Input: part model. Units: mm. Frame: model coordinates. A direction names the side the tool comes from. Round coordinates to 2 decimals unless told otherwise and drop trailing zeros. Loops run counter-clockwise (first coordinate to the right, second up) from the corner with the lowest first, then second, coordinate; pieces in that order, holes last. Notation, with made-up numbers: (3.5, -24.5) -> (36.5, -24.5) arc R19 ccw to (36.5, -10.5) -> close; hole circle Ø4 at (45.25, -19). An arc over 180 degrees is marked (long way). Answer as a JSON object with one key per item and string values. Group by question number.
Item 1: Section query B-B on z = 10. Return loops of the section in (x, y).
Item 2: Section query A-A on x = 0. Return loops of the section in (y, z), and give its area (3 significant figures).
Item 3: Section query C-C on y = -14. Return loops of the section in (x, z), and give its area (3 significant figures).
Item 4: Set-up query: faces 4 (the cylindrical face through (0.51, -74.23, -8.38)), 5 (the flat face through (-2, 72.2, 9)), 6 (the flat face through (-2, -72.2, -9)). Return all of +Z, -Z, +X, -X, +Y, -Y with unobstructed straight access to the full face (end or side cutting, diameter ignored); none if empty.
Item 5: Pin query (flat end, axial travel): pin 1 (1 mm diameter, centred on x = 5.5, y = -6.5, fed in from +Z); pin 2 (2.5 mm diameter, centred on x = -0.5, z = 9.5, fed in from +Y); pin 3 (5 mm diameter, centred on x = -4.5, y = -27, fed in from -Z). Return the tip coordinate at first contact, or that it passes through.
Item 6: Material intervals for line 1 (Y direction, x = 3.5, z = 7.75); line 2 (X direction, y = 74.35, z = 10); line 3 (Z direction, x = -0.25, y = -47), sorted ascending. Write a range as [from, to].
Item 7: Draft query along Z for faces 1 (the flat face through (0, -74, -13.75)), 2 (the cylindrical face through (-1.66, 74.23, 9.63)), 3 (the flat face through (-7, 0, 1)). Return one class per face: released by +Z, released by -Z, zero draft, split by the parting line, or undercut.
from build123d import *

# Parameters (mm, degrees)
SKETCH1_W           = 14
SKETCH1_H           = 10
BOSS_EXTRUDE1_DEPTH = 76.2
SKETCH3_W           = 14
SKETCH3_H           = 27.5
SKETCH3_R           = 1.7
BOSS_EXTRUDE3_DEPTH = 4


with BuildPart() as part:
    # Sketch1 → Boss-Extrude1 (new, symmetric)
    with BuildSketch(Plane(origin=(0, 0, 0), x_dir=(1, 0, 0), z_dir=(0, 1, 0))):
        Rectangle(SKETCH1_W, SKETCH1_H)
    extrude(amount=BOSS_EXTRUDE1_DEPTH, both=True)

    # Sketch3 → Boss-Extrude3 (add)
    with BuildSketch(Plane(origin=(0, 76.2, 0), x_dir=(1, 0, 0), z_dir=(0, 1, 0))):
        Rectangle(SKETCH3_W, SKETCH3_H)
        with Locations(Location((0, 10, 0), (0, 0, 270))):
            Circle(SKETCH3_R, mode=Mode.SUBTRACT)
        with Locations(Location((0, -10, 0), (0, 0, 270))):
            Circle(SKETCH3_R, mode=Mode.SUBTRACT)
    boss_extrude3 = extrude(amount=-BOSS_EXTRUDE3_DEPTH)

    # Mirror1: Boss-Extrude3 across plane
    add(boss_extrude3.mirror(Plane.ZX))


solid = part.part
Solved:
{
 "1": {"outline": "(-7, -76.2) -> (-1.7, -76.2) -> (-1.7, -72.2) -> (-7, -72.2) -> close; (-7, 72.2) -> (-1.7, 72.2) -> (-1.7, 76.2) -> (-7, 76.2) -> close; (1.7, -76.2) -> (7, -76.2) -> (7, -72.2) -> (1.7, -72.2) -> close; (1.7, 72.2) -> (7, 72.2) -> (7, 76.2) -> (1.7, 76.2) -> close"},
 "2": {"outline": "(-76.2, -13.75) -> (-72.2, -13.75) -> (-72.2, -11.7) -> (-76.2, -11.7) -> close; (-76.2, -8.3) -> (-72.2, -8.3) -> (-72.2, -5) -> (72.2, -5) -> (72.2, -8.3) -> (76.2, -8.3) -> (76.2, 8.3) -> (72.2, 8.3) -> (72.2, 5) -> (-72.2, 5) -> (-72.2, 8.3) -> (-76.2, 8.3) -> close; (-76.2, 11.7) -> (-72.2, 11.7) -> (-72.2, 13.75) -> (-76.2, 13.75) -> close; (72.2, -13.75) -> (76.2, -13.75) -> (76.2, -11.7) -> (72.2, -11.7) -> close; (72.2, 11.7) -> (76.2, 11.7) -> (76.2, 13.75) -> (72.2, 13.75) -> close", "area": "1,610 mm²"},
 "3": {"outline": "(-7, -5) -> (7, -5) -> (7, 5) -> (-7, 5) -> close", "area": "140 mm²"},
 "4": {"face 4": "+Y, -Y", "face 5": "+Z, +X, -X", "face 6": "-Z, +X, -X"},
 "5": {"pin 1": "z = 5", "pin 2": "y = 76.2", "pin 3": "z = -5"},
 "6": {"line 1": "[-76.2, -72.2], [72.2, 76.2]", "line 2": "[-7, -1.7], [1.7, 7]", "line 3": "[-5, 5]"},
 "7": {"face 1": "released by -Z", "face 2": "undercut", "face 3": "zero draft"}
}
